from build123d import *

# Parameters (mm, degrees)
F0_W     = 152.908
F0_H     = 159.004
F1_DEPTH = 6.35
F2_DEPTH = 12.7
F3_R     = 1.905
F4_DEPTH = 6.35
F0_W_2   = 3.047997
F5_DEPTH = 6.35


with BuildPart() as f1:
    # F0 (on Top) → F1 (new body)
    with BuildSketch(Plane.XY):
        Rectangle(F0_W, F0_H)
    extrude(amount=F1_DEPTH)

    # F0 (on Top) → F2 (join)
    with BuildSketch(Plane.XY):
        Polygon((79.501997, -79.502), (76.454, -79.502), (-76.454, -79.502), (-76.454, 79.502), (76.454, 79.502), (79.501997, 79.502), (79.501997, 82.549997), (-79.501997, 82.549997), (-79.501997, -82.549997), (79.501997, -82.549997), align=None)
    extrude(amount=F2_DEPTH)

    # F3 (on face) → F4 (join)
    with BuildSketch(Plane.YZ.offset(76.454)):
        with Locations((-63.078232, 3.175)):
            Circle(F3_R)
        with Locations((-22.438232, 3.175)):
            Circle(F3_R)
        with Locations((18.201768, 3.175)):
            Circle(F3_R)
        with Locations((58.841768, 3.175)):
            Circle(F3_R)
    extrude(amount=F4_DEPTH)

    # F0 (on Top) → F5 (join)
    with BuildSketch(Plane.XY):
        with Locations((77.977998, 0)):
            Rectangle(F0_W_2, F0_H)
    extrude(amount=F5_DEPTH)


solid = f1.part
Can you work these out from the model? Positions are in its coordinate system, mm. A direction names the side the tool comes from. Coordinates: 2 decimals unless noted, no trailing zeros. Loops run counter-clockwise (first coordinate to the right, second up) from the corner with the lowest first, then second, coordinate; pieces in that order, holes last. Notation, with made-up numbers: (2, 48) - (26, 48) arc R36 ccw to (26, 86) - close; hole circle Ø11 at (31.25, 47). An arc over 180 degrees is marked (long way). Answer as a JSON object with one key per item and string values. Group by question number.
Item 1: If I drill on L1, parallel to Y at x = -49.5, z = 9.5; L2, parallel to X at y = -27, z = 7; L3, parallel to X at y = -44.5, z = 1.75, over which ranges is the centre line in solid material (lowest first)? Write a range as from..to.
Item 2: On a 3-axis mill with a long thin cutter (end or side, diameter ignored), from which of +Z, -Z, +X, -X, +Y, -Y can I reach the whole of each face in a straight line? I mean faces 5 (the face through (0, 1, 6.35)), 6 (the face through (81.13, -20.62, 3.75)), 7 (the face through (-77, 37, 12.7)). Say none if no direction works.
Item 3: If we section it at B-B (x = 57.5): List the corners of the cut face in (y, z) for me.
Item 4: If we mould it in two halves opening along Y, with no side actions, what happens to faces 1 (the face through (-1, -82.55, 6)), 2 (the face through (3, -79.502, 9)), 3 (the face through (82.804, 18, 3)), 4 (the face through (0, 79.502, 9))? For each: released by +Y, released by -Y, zero draft, split by the parting line, or undercut.
Item 5: If we section it at C-C (y = 29): List the corners of the cut face in (x, z) for me.
Item 6: For pin 1 (0.9 mm diameter, centred on y = 80.5, z = 6, fed in from +X); pin 2 (6 mm diameter, centred on x = -6.5, y = 44, fed in from +Z); pin 3 (1.9 mm diameter, centred on y = -8.5, z = 8, fed in from +X), each with a flat end and sliding along its axis, tell me the tip position at first contact or that it passes through.
Item 7: If we section it at A-A (z = 9.5): List the corners of the cut face in (x, y) for me.
Returned:
{
 "1": {"L1": "y = -82.55..-79.5, 79.5..82.55", "L2": "x = -79.5..-76.45", "L3": "x = -79.5..79.5"},
 "2": {"face 5": "+Z, +X", "face 6": "+X", "face 7": "+Z, +X, -X, +Y, -Y"},
 "3": {"outline": "(-82.55, 0) - (82.55, 0) - (82.55, 12.7) - (79.5, 12.7) - (79.5, 6.35) - (-79.5, 6.35) - (-79.5, 12.7) - (-82.55, 12.7) - close"},
 "4": {"face 1": "released by -Y", "face 2": "undercut", "face 3": "zero draft", "face 4": "undercut"},
 "5": {"outline": "(-79.5, 0) - (79.5, 0) - (79.5, 6.35) - (-76.45, 6.35) - (-76.45, 12.7) - (-79.5, 12.7) - close"},
 "6": {"pin 1": "stops at x = 79.5", "pin 2": "stops at z = 6.35", "pin 3": "stops at x = -76.45"},
 "7": {"outline": "(-79.5, -82.55) - (79.5, -82.55) - (79.5, -79.5) - (-76.45, -79.5) - (-76.45, 79.5) - (79.5, 79.5) - (79.5, 82.55) - (-79.5, 82.55) - close"}
}
